Geometry: final body of the model. Coordinates: model frame, mm. A direction names the side the tool comes from. Give positions to 0.01 mm unless a question says otherwise; leave off trailing zeros. Write each loop counter-clockwise with the first axis right and the second up, starting at its lowest first coordinate (ties: lowest second). Pieces come first, ordered by that corner, then holes.
Q1. Line query: L1, parallel to X at y = -8, z = 12; L2, parallel to X at y = -6.25, z = 15; L3, parallel to Z at x = 38, y = -22.5. Output: solid intervals per line, ascending.
Q2. Pin query (flat end, axial travel): pin 1 (3 mm diameter, centred on y = 26, z = 68.5, fed in from +X); pin 2 (10 mm diameter, centred on y = 19.5, z = 65, fed in from +X); pin 3 (6 mm diameter, centred on x = 44, y = -5.5, fed in from +Z); pin 4 (13.5 mm diameter, centred on x = -55.24, z = 15, fed in from +Y) (3 decimals). Return the tip coordinate at first contact, or that it passes through.
Q3. Reachability of faces 4 (the face through (-51, -12, 0)), 5 (the face through (-4, -40, 0)), 6 (the face through (15, 23, 75)), 7 (the face through (51, -10, 0)) from +Z, -Z, +X, -X, +Y, -Y: full face, straight path, thin tool, end or side. Return the list, or none.
Q4. Cut plane D-D on z = 81.5. Return the cut outline in (x, y).
Q5. Draft query along Y for faces 1 (the face through (5.21, -39.66, 44.37)), 2 (the face through (-3.955, 30.9, 9.842)), 3 (the face through (-0.513, -39.195, -1.376)). Return one class per face: pulls with the +Y half, pulls with the -Y half, needs draft (parallel to the pull), parting line crosses it, or undercut.
Q6. Cut plane B-B on x = 59.5. Return the cut outline in (y, z).
Q7. Cut plane A-A on y = 13.5. Return the cut outline in (x, z).
Q8. Cut plane C-C on y = -9.5. Return the cut outline in (x, z).
```python
from build123d import *

# Parameters (mm, degrees)
BOSS_EXTRUDE1_DEPTH       = 90
BOSS_EXTRUDE2_START       = -20
BOSS_EXTRUDE2_DEPTH       = 20
SKETCH3_R                 = 7.5
BOSS_EXTRUDE9_DEPTH       = 20
CUT_EXTRUDE1_REACH        = 147.378
CUT_EXTRUDE1_END_RADIUS   = 22.5
SKETCH5_R                 = 6.5
SKETCH5_3_W               = 40
SKETCH5_3_H               = 100
CUT_EXTRUDE2_DEPTH        = 10
F_2_0MM_DOWEL_HOLE1_D     = 11
F_2_0MM_DOWEL_HOLE1_DEPTH = 16
F_2_0MM_DOWEL_HOLE1_TIP   = 3.175426481


with BuildPart() as part:
    # Sketch1 → Boss-Extrude1 (new body)
    with BuildSketch(Plane.XY):
        with BuildLine():
            ThreePointArc((40, 0), (0, 40), (-40, 0))
            Line((-40, 0), (-30, 0))
            ThreePointArc((-30, 0), (0, 30), (30, 0))
            Line((30, 0), (40, 0))
        make_face()
        with BuildLine():
            Line((-30, 0), (-40, 0))
            ThreePointArc((-40, 0), (0, -40), (40, 0))
            Line((40, 0), (30, 0))
            ThreePointArc((30, 0), (0, -30), (-30, 0))
        make_face()
        with BuildLine():
            ThreePointArc((30, 0), (0, 30), (-30, 0))
            Line((-30, 0), (-22.5, 0))
            ThreePointArc((-22.5, 0), (0, 22.5), (22.5, 0))
            Line((22.5, 0), (30, 0))
        make_face()
        with BuildLine():
            Line((-22.5, 0), (-30, 0))
            ThreePointArc((-30, 0), (0, -30), (30, 0))
            Line((30, 0), (22.5, 0))
            ThreePointArc((22.5, 0), (0, -22.5), (-22.5, 0))
        make_face()
    extrude(amount=BOSS_EXTRUDE1_DEPTH)

    # Sketch1_3 → Boss-Extrude2 (add)
    with BuildSketch(Plane.XY.offset(BOSS_EXTRUDE2_START)):
        with BuildLine():
            Line((-40, 0), (-50, 0))
            ThreePointArc((-50, 0), (0, -50), (50, 0))
            Line((50, 0), (40, 0))
            ThreePointArc((40, 0), (0, -40), (-40, 0))
        make_face()
        with BuildLine():
            Line((-30, 0), (-40, 0))
            ThreePointArc((-40, 0), (0, -40), (40, 0))
            Line((40, 0), (30, 0))
            ThreePointArc((30, 0), (0, -30), (-30, 0))
        make_face()
    extrude(amount=BOSS_EXTRUDE2_DEPTH)

    # Sketch3 → Boss-Extrude9 (add)
    # profile 1 of 2: a face of its own
    with BuildSketch(Plane(origin=(0, 0, 0), x_dir=(1, 0, 0), z_dir=(0, 1, 0))):
        with BuildLine():
            Line((34.445197512, 0), (55, 0))
            ThreePointArc((55, 0), (70.244929467, -14.755070533), (55.489858934, -30))
            Line((55.489858934, -30), (34.445197512, -30))
            Line((34.445197512, -30), (34.445197512, 0))
        make_face()
        with Locations(Location((55.244929467, -15, 0), (0, 0, 270))):
            Circle(SKETCH3_R, mode=Mode.SUBTRACT)
    # profile 2 of 2: a face of its own
    with BuildSketch(Plane(origin=(0, 0, 0), x_dir=(1, 0, 0), z_dir=(0, 1, 0))):
        with BuildLine():
            Line((-34.445197512, 0), (-34.445197512, -30))
            Line((-34.445197512, -30), (-55.489858934, -30))
            ThreePointArc((-55.489858934, -30), (-70.244929467, -14.755070533), (-55, 0))
            Line((-55, 0), (-34.445197512, 0))
        make_face()
        with Locations(Location((-55.244929467, -15, 0), (0, 0, 270))):
            Circle(SKETCH3_R, mode=Mode.SUBTRACT)
    extrude(amount=-BOSS_EXTRUDE9_DEPTH)

    # Cut-Extrude1: up to this cylinder (the profile starts outside it)
    cut_extrude1_end = Plane(origin=(0, 0, 41.9876885), z_dir=(0, 0, -1)) * Cylinder(CUT_EXTRUDE1_END_RADIUS, 394.731377, mode=Mode.PRIVATE)
    # Sketch5 → Cut-Extrude1 (cut, up to the surface)
    with BuildSketch(Plane(origin=(0, 40, 0), x_dir=(1, 0, 0), z_dir=(0, 1, 0)), mode=Mode.PRIVATE) as cut_extrude1_sk1:
        with BuildLine():
            Line((15, -60), (15, -90))
            Line((15, -90), (-15, -90))
            Line((-15, -90), (-15, -60))
            ThreePointArc((-15, -60), (0, -45), (15, -60))
        make_face()
    cut_extrude1_tool1 = extrude(cut_extrude1_sk1.sketch, amount=-CUT_EXTRUDE1_REACH, mode=Mode.PRIVATE) - cut_extrude1_end
    add(cut_extrude1_tool1.solids().sort_by_distance((0, 40, 68.975377))[0], mode=Mode.SUBTRACT)
    # Sketch5 → Cut-Extrude1 (cut, up to the surface)
    with BuildSketch(Plane(origin=(0, 40, 0), x_dir=(1, 0, 0), z_dir=(0, 1, 0)), mode=Mode.PRIVATE) as cut_extrude1_sk2:
        with Locations(Location((0, -15, 0), (0, 0, 270))):
            Circle(SKETCH5_R)
    cut_extrude1_tool2 = extrude(cut_extrude1_sk2.sketch, amount=-CUT_EXTRUDE1_REACH, mode=Mode.PRIVATE) - cut_extrude1_end
    add(cut_extrude1_tool2.solids().sort_by_distance((0, 40, 15))[0], mode=Mode.SUBTRACT)

    # Sketch5_3 → Cut-Extrude2 (cut)
    with BuildSketch(Plane(origin=(0, 40, 0), x_dir=(1, 0, 0), z_dir=(0, 1, 0))):
        with Locations((0, -90)):
            Rectangle(SKETCH5_3_W, SKETCH5_3_H)
        with BuildLine():
            ThreePointArc((15, -60), (0, -45), (-15, -60))
            Line((-15, -60), (-15, -90))
            Line((-15, -90), (15, -90))
            Line((15, -90), (15, -60))
        make_face(mode=Mode.SUBTRACT)
    extrude(amount=-CUT_EXTRUDE2_DEPTH, mode=Mode.SUBTRACT)

    # 2.0mm Dowel Hole1
    with Locations(Plane(origin=(0, 0, -20), x_dir=(-1, 0, 0), z_dir=(0, 0, -1))):
        with Locations((0, -40)):
            Hole(F_2_0MM_DOWEL_HOLE1_D / 2, depth=F_2_0MM_DOWEL_HOLE1_DEPTH)
            with Locations((0, 0, -(F_2_0MM_DOWEL_HOLE1_DEPTH + F_2_0MM_DOWEL_HOLE1_TIP / 2))):  # 120° drill point
                Cone(0, F_2_0MM_DOWEL_HOLE1_D / 2, F_2_0MM_DOWEL_HOLE1_TIP, mode=Mode.SUBTRACT)


solid = part.part
```
Data:
1. L1: x = -69.94 to -62.12, -48.37 to -21.03, 21.03 to 48.37, 62.12 to 69.94
1. L2: x = -70.25 to -62.74, -47.74 to -21.61, 21.61 to 47.74, 62.74 to 70.25
1. L3: z = -20 to 0
2. pin 1: stops at x = 31.62
2. pin 2: stops at x = 37.28
2. pin 3: stops at z = 30
2. pin 4: passes through
3. face 4: -Z, -X, -Y
3. face 5: +Z, -Y
3. face 6: +Z, +Y
3. face 7: -Z, +X, -Y
4. outline: (-20, 30) - (-20, 34.64) arc R40 ccw (long way) to (20, 34.64) - (20, 30) - (15, 30) - (15, 16.77) arc R22.5 cw (long way) to (-15, 16.77) - (-15, 30) - close
5. face 1: parting line crosses it
5. face 2: needs draft
5. face 3: undercut
6. outline: (-20, 0.61) - (0, 0.61) - (0, 8.82) - (-20, 8.82) - close; (-20, 21.18) - (0, 21.18) - (0, 29.39) - (-20, 29.39) - close
7. outline: (-37.65, 0) - (-18, 0) - (-18, 90) - (-37.65, 90) - close; (18, 0) - (37.65, 0) - (37.65, 90) - (18, 90) - close
8. outline: (-55.49, 30) arc R15 ccw to (-55, 0) - (-49.09, 0) - (-49.09, -20) - (-28.46, -20) - (-28.46, 0) - (-20.4, 0) - (-20.4, 90) - (-38.86, 90) - (-38.86, 30) - close; (20.4, 0) - (28.46, 0) - (28.46, -20) - (49.09, -20) - (49.09, 0) - (55, 0) arc R15 ccw to (55.49, 30) - (38.86, 30) - (38.86, 90) - (20.4, 90) - close; hole circle Ø15 at (-55.24, 15); hole circle Ø15 at (55.24, 15)
